Geometry check sheet. Reference: the model listing, model coordinates, mm. Face numbers are marked on the shaded views. A direction names the side the tool comes from. Coordinates: 2 decimals unless noted, no trailing zeros. Loops run counter-clockwise (first coordinate to the right, second up) from the corner with the lowest first, then second, coordinate; pieces in that order, holes last.
from build123d import *

# Parameters (mm, degrees)
F0_W     = 38.1
F0_H     = 31.75
F0_R     = 6.35
F1_DEPTH = 3.175
F2_W     = 38.1
F2_H     = 3.175
F3_DEPTH = 50.8
F4_R     = 3.175
F5_DEPTH = 3.176


with BuildPart() as f1:
    # F0 (on Front) → F1 (new body)
    with BuildSketch(Plane.XZ):
        with Locations((19.05, 15.875)):
            Rectangle(F0_W, F0_H)
        with Locations((19.05, 15.875)):
            Circle(F0_R, mode=Mode.SUBTRACT)
    extrude(amount=F1_DEPTH)

    # F2 (on face) → F3 (join)
    with BuildSketch(Plane(origin=(0, 0, 0), x_dir=(-1, 0, 0), z_dir=(0, 1, 0))):
        with Locations((-19.05, 1.5875)):
            Rectangle(F2_W, F2_H)
    extrude(amount=F3_DEPTH)

    # F4 (on face) → F5 (cut, through all)
    with BuildSketch(Plane.XY.offset(3.175)):
        with Locations((28.575, 25.4)):
            Circle(F4_R)
        with Locations((9.525, 25.4)):
            Circle(F4_R)
    extrude(amount=-F5_DEPTH, mode=Mode.SUBTRACT)


solid = f1.part
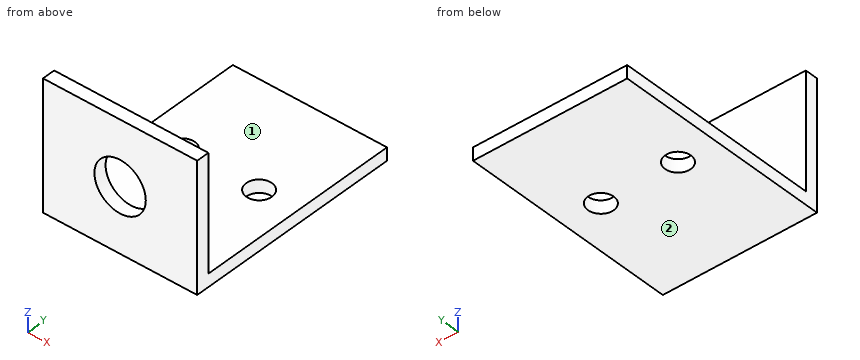
(1) Scan lines: L1, parallel to Z at x = 17, y = 17 (3 decimals); L2, parallel to Y at x = 3, z = 25.5 (3 decimals). Record each from-to range of solid material in increasing order.
Findings:
L1: z = 0 to 3.175
L2: y = -3.175 to 0
(2) Access from +Z, -Z, +X, -X, +Y, -Y to the whole of each face (thin tool, end or side, straight path). Record for the marked faces 1 and 2.
Findings:
face 1: +Z, +X, -X, +Y
face 2: -Z, +X, -X, +Y, -Y
(3) Sectioned sample at B-B on y = 25.4. Record the cut outline in (x, z) (3 decimals), and give its area (3 significant figures).
Findings:
outline: (0, 0) - (6.35, 0) - (6.35, 3.175) - (0, 3.175) - close; (12.7, 0) - (25.4, 0) - (25.4, 3.175) - (12.7, 3.175) - close; (31.75, 0) - (38.1, 0) - (38.1, 3.175) - (31.75, 3.175) - close
area: 80.6 mm2
(4) Sectioned sample at A-A on x = 19.05. Record the cut outline in (y, z) (3 decimals), and give its area (3 significant figures).
Findings:
outline: (-3.175, 0) - (50.8, 0) - (50.8, 3.175) - (0, 3.175) - (0, 9.525) - (-3.175, 9.525) - close; (-3.175, 22.225) - (0, 22.225) - (0, 31.75) - (-3.175, 31.75) - close
area: 222 mm2
(5) Sectioned sample at D-D on x = 5. Record the cut outline in (y, z) (3 decimals), and give its area (3 significant figures).
Findings:
outline: (-3.175, 0) - (50.8, 0) - (50.8, 3.175) - (0, 3.175) - (0, 31.75) - (-3.175, 31.75) - close
area: 262 mm2
(6) Gauge pin test, flat ends, axial feed: pin 1 Ø8 at (x, y) = (28, 43.5) entering from -Z; pin 2 Ø11.5 at (x, y) = (19, 30) entering from +Z (3 decimals); pin 3 Ø8.5 at (x, z) = (28, 11) entering from +Y. Record the tip position at first contact, or that the pin passes through.
Findings:
pin 1: stops at z = 0
pin 2: stops at z = 3.175
pin 3: stops at y = 0
(7) Sectioned sample at C-C on z = 18. Record the cut outline in (x, y) (3 decimals), and give its area (3 significant figures).
Findings:
outline: (0, -3.175) - (13.066, -3.175) - (13.066, 0) - (0, 0) - close; (25.034, -3.175) - (38.1, -3.175) - (38.1, 0) - (25.034, 0) - close
area: 83.0 mm2
